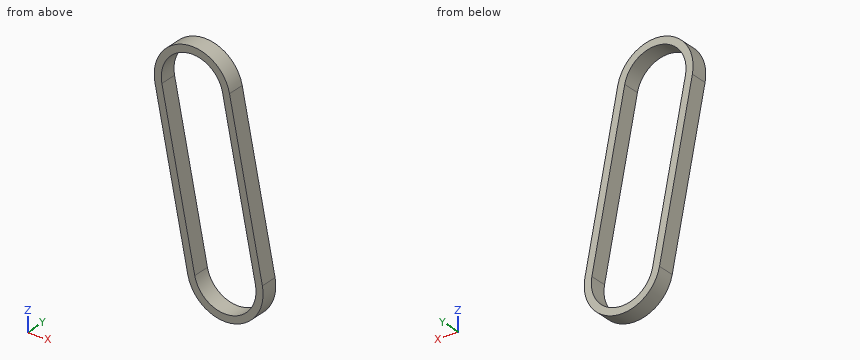
```python
from build123d import *

# Parameters (mm, degrees)
BOSS_EXTRUDE1_DEPTH = 4.5


with BuildPart() as part:
    # Sketch1 → Boss-Extrude1 (new, symmetric)
    with BuildSketch(Plane(origin=(0, 254.392577481, 0), x_dir=(1, 0, 0), z_dir=(0, 1, 0))):
        with BuildLine():
            Line((25.484273554, -181.693777747), (7.854508283, -269.943103479))
            ThreePointArc((7.854508283, -269.943103479), (-16.146601218, -285.951437018), (-32.154934757, -261.950327517))
            Line((-32.154934757, -261.950327517), (-14.525169486, -173.701001785))
            ThreePointArc((-14.525169486, -173.701001785), (9.475940015, -157.692668245), (25.484273554, -181.693777747))
        make_face()
        with BuildLine():
            ThreePointArc((21.757903859, -180.949352535), (8.731514803, -161.41903794), (-10.798799791, -174.445426997))
            Line((-10.798799791, -174.445426997), (-28.428565062, -262.694752729))
            ThreePointArc((-28.428565062, -262.694752729), (-15.402176006, -282.225067323), (4.128138588, -269.198678267))
            Line((4.128138588, -269.198678267), (21.757903859, -180.949352535))
        make_face(mode=Mode.SUBTRACT)
    extrude(amount=BOSS_EXTRUDE1_DEPTH, both=True)


solid = part.part
```
Geometry check sheet. Reference: the model listing, model coordinates, mm. Round coordinates to 2 decimals unless told otherwise and drop trailing zeros. Loops run counter-clockwise (first coordinate to the right, second up) from the corner with the lowest first, then second, coordinate; pieces in that order, holes last. Notation, with made-up numbers: (27, -6.5) - (75, -6.5) arc R14 ccw to (75, 13.5) - close; hole circle Ø8 at (-7, 86.25). An arc over 180 degrees is marked (long way). Use a Markdown table: item, result.
Q1. Cross-section at C-C on z = 197.5. Record the cut outline in (x, y), plus the area to 3 significant figures.
Solutions:
| item | result |
|---|---|
| outline | (-19.28, 249.89) - (-15.4, 249.89) - (-15.4, 258.89) - (-19.28, 258.89) - close; (18.45, 249.89) - (22.33, 249.89) - (22.33, 258.89) - (18.45, 258.89) - close |
| area | 69.8 mm2 |
Q2. Cross-section at A-A on x = -19.5. Record the cut outline in (y, z).
Solutions:
| item | result |
|---|---|
| outline | (249.89, 198.6) - (258.89, 198.6) - (258.89, 218) - (249.89, 218) - close; (249.89, 280.83) - (258.89, 280.83) - (258.89, 284.98) - (249.89, 284.98) - close |
Q3. Material ranges on line 1 (X direction, y = 251, z = 176); line 2 (Z direction, x = -2, y = 253); line 3 (Z direction, x = -6, y = 252), recorded low to high.
Solutions:
| item | result |
|---|---|
| line 1 | x = -14.98 to -11.11, 21.99 to 25.81 |
| line 2 | z = 158.72 to 162.88, 279.08 to 283.64 |
| line 3 | z = 160.83 to 165.71, 281.37 to 285.4 |
Q4. Go/stop test with flat-tipped pins: P1, Ø1.5, axis at x = -21.5, y = 251.5, coming from the +Z side; P2, Ø3, axis at x = -16.5, z = 211, coming from the -Y side; P3, Ø3, axis at y = 254.5, z = 265.5, coming from the +X side; P4, Ø3, axis at y = 257, z = 198.5, coming from the -X side. Record where each tip stops, or that it passes through.
Solutions:
| item | result |
|---|---|
| P1 | stops at z = 284.45 |
| P2 | passes through |
| P3 | stops at x = 9.04 |
| P4 | stops at x = -19.78 |
